Could you check a few things on this model? Use its own coordinates, in mm. A direction names the side the tool comes from. Give positions to 0.01 mm unless a question says otherwise; leave off trailing zeros. Order: outer loops, then holes, each group sorted by start corner. A loop starts at its lowest first (then second) coordinate and runs counter-clockwise, first axis right, second up. Notation, with made-up numbers: (73.25, 16.25) -> (114.25, 16.25) arc R16 cw to (114.25, 21.25) -> close; hole circle Ø6 at (-19.75, 75). An arc over 180 degrees is marked (long way). Answer as CSV lines item,"result". Start each with the question number.
(1) I want a section at A-A (z = -1). Please give me the cut outline in (x, y), plus the area to 3 significant figures.
(2) We'd pull the mould along Y, two halves only. Please class faces 4 (the face through (-6, 1, -2)), 5 (the face through (-0.6, 2.57, -1.48)), 6 (the face through (0, 2, -1)), 7 (the face through (-9.43, 2.6, -1.48)): released by +Y, released by -Y, zero draft, split by the parting line, or undercut.
(3) On a 3-axis mill with a long thin cutter (end or side, diameter ignored), from which of +Z, -Z, +X, -X, +Y, -Y can I reach the whole of each face in a straight line? I mean faces 1 (the face through (-10, 5, -2)), 2 (the face through (-7, 2, -2)), 3 (the face through (0, 5, -1)). Say none if no direction works.
(4) I want a section at D-D (y = 9.5). Please give me the cut outline in (x, z).
(5) I want a section at C-C (x = 0.5). Please give me the cut outline in (y, z), plus the area to 3 significant figures.
(6) I need wall thicknesses on L1, parallel to X at y = 7, z = -0.6; L2, parallel to Y at x = -5, z = -2.1; L3, parallel to Y at x = 0.5, z = -2.05. Which ranges of each line are inside material? Lowest first, please.
(7) Will these pins go through, and if not, where does the flat tip stop? pin 1 Ø2 at (x, y) = (-5, 7) entering from +Z; pin 2 Ø1 at (x, z) = (-4, -2) entering from +Y; pin 3 Ø1.5 at (y, z) = (5.5, -1) entering from +X; pin 4 Ø1.6 at (x, z) = (-7, -1) entering from -Y.
(8) I want a section at B-B (x = -5). Please give me the cut outline in (y, z).
Autodesk Inventor part; units mm, degrees
ref_plane "YZ Plane" through (0, 0, 0) normal (1, 0, 0) x (0, 1, 0)
ref_plane "XZ Plane" through (0, 0, 0) normal (0, 1, 0) x (-1, 0, 0)
ref_plane "XY Plane" through (0, 0, 0) normal (0, 0, 1) x (1, 0, 0)
sketch "Sketch1" plane through (0, 0, 0) normal (0, 1, 0) x (-1, 0, 0)
  line L0 (0, 0) -> (0, -3)
  line L1 (0, -3) -> (10, -3)
  line L2 (10, -3) -> (10, 0)
  line L3 (10, 0) -> (0, 0)
  dimension "d0" = 3
  dimension "d1" = 10
  dimension "d2" = 90
  dimension "d3" = 3
extrude "Extrusion1" add sketch "Sketch1" along normal blind 12
sketch "Sketch4" plane through (0, 0, -3) normal (0, 0, -1) x (-1, 0, 0)
  line L0 (0, 0) -> (0, 2)
  line L1 (0, 0) -> (0, 12)
  line L2 (0, 2) -> (4, 2)
  line L3 (10, 0) -> (10, 12)
  line L4 (4, 2) -> (0, 0)
  line L5 (0, 0) -> (10, 0)
  line L6 (10, 0) -> (10, 2)
  line L7 (10, 2) -> (6, 2)
  line L8 (6, 2) -> (10, 0)
  line L9 (4, 2) -> (6, 2)
  line L10 (6, 2) -> (6, 0)
  line L11 (4, 2) -> (4, 0)
  line L12 (4, 0) -> (6, 0)
  dimension "d9" = 2
  dimension "d10" = 4
  dimension "d11" = 2
  dimension "d12" = 4
extrude "Extrusion3" cut sketch "Sketch4" against normal up to surface (3 mm away) contours L0 L2 L4 | L4 L11 L5 | L7 L3 L8 | L8 L5 L10
sketch "Sketch6" plane through (0, 12, -3) normal (0, 0, -1) x (-1, 0, 0)
  line L0 (0, -10) -> (0, 0)
  line L1 (0, -5) -> (10, -5)
  line L2 (10, -10) -> (10, 0)
  line L3 (0, 0) -> (10, 0)
  line L4 (5, 0) -> (5, -10)
  circle A0 centre (5, -5) radius 1.75
  point P0 (0, -12)
  dimension "d15" = 3.5
extrude "Extrusion4" cut sketch "Sketch6" against normal up to surface (3 mm away) contours A0 L4 L1 | L1 L4 A0 | L4 A0 L1 | L1 A0 L4
fillet "Fillet1" radius 2 4 edges at (0, 12, -1.5) (0, 2, -1.5) (-10, 12, -1.5) (-10, 2, -1.5)
sketch "Sketch7" plane through (-8, 12, 0) normal (0, 0, 1) x (1, 0, 0)
  circle A0 centre (3, -5) radius 1.75
  arc A1 (8, -2) -> (6, 0) centre (6, -2) ccw
  circle A2 centre (3, -5) radius 5
  line L0 (6, 0) -> (0, 0)
  line L1 (2, -12) -> (4, -12)
  line L2 (4, -10) -> (6, -10)
  arc A3 (6, -10) -> (8, -8) centre (6, -8) ccw
  line L3 (8, -8) -> (8, -2)
  arc A4 (8, -2) -> (6, 0) centre (6, -2) ccw
  line L4 (0, 0) -> (6, 0)
  arc A5 (0, 0) -> (-2, -2) centre (0, -2) ccw
  line L5 (-2, -8) -> (-2, -2)
  arc A6 (-2, -8) -> (0, -10) centre (0, -8) ccw
  line L6 (0, -10) -> (2, -10)
  circle A7 centre (3, -5) radius 1.75
  line L7 (2, -10) -> (2, -12)
  line L8 (4, -12) -> (4, -10)
  point P0 (8, -12)
  point P1 (-2, -5)
  point P2 (3, 0)
  point P3 (8, -5)
  point P4 (8, -2)
extrude "Extrusion5" cut sketch "Sketch7" against normal up to surface (3 mm away) contours L3 A2 L0 A1 | A2 L5 A5 L0
sketch "Sketch8" plane through (-4, 0, -3) normal (1, 0, 0) x (0, 0, -1)
  line L0 (0, 2) -> (0, 0)
  line L1 (-3, 0) -> (-3, 2)
  line L2 (0, 0) -> (-3, 0)
  line L3 (-3, 0) -> (-3, 2)
  line L4 (-3, 2) -> (0, 2)
  line L5 (0, 2) -> (0, 0)
extrude "Extrusion6" add sketch "Sketch8" along normal blind 7
properties part number "Knuckle Attachment SMALL HOLE"
Final values:
1,outline,"(-10, 4) arc R2 ccw to (-8, 2) -> (-6, 2) -> (-6, 0) -> (3, 0) -> (3, 2) -> (-2, 2) arc R2 ccw to (0, 4) -> (0, 7) arc R5 ccw to (-10, 7) -> close; hole circle Ø3.5 at (-5, 7)"
1,area,"95.9 mm²"
2,face 4,"zero draft"
2,face 5,"undercut"
2,face 6,"undercut"
2,face 7,"released by -Y"
3,face 1,"+Z, -Z, -X, +Y, -Y"
3,face 2,"+Z, -Z, -X, -Y"
3,face 3,"+Z, -Z, +X, +Y"
4,outline,"(-9.33, -3) -> (-0.67, -3) -> (-0.67, 0) -> (-9.33, 0) -> close"
5,outline,"(0, -3) -> (2, -3) -> (2, 0) -> (0, 0) -> close"
5,area,"6.00 mm²"
6,L1,"-10 to -6.75, -3.25 to 0"
6,L2,"0 to 5.25, 8.75 to 12"
6,L3,"0 to 2"
7,pin 1,"through"
7,pin 2,"y = 11.97"
7,pin 3,"x = 0"
7,pin 4,"y = 2"
8,outline,"(0, -3) -> (5.25, -3) -> (5.25, 0) -> (0, 0) -> close; (8.75, -3) -> (12, -3) -> (12, 0) -> (8.75, 0) -> close"
